The figure shows three views and two pictorial views of one solid part (mm, origin at its lowest corner). Answer the questions. A direction names the side the tool comes from. Coordinates: 2 decimals unless noted, no trailing zeros. Write each loop counter-clockwise with the first axis right and the second up, starting at its lowest first coordinate (ties: lowest second). Pieces come first, ordered by that corner, then holes.
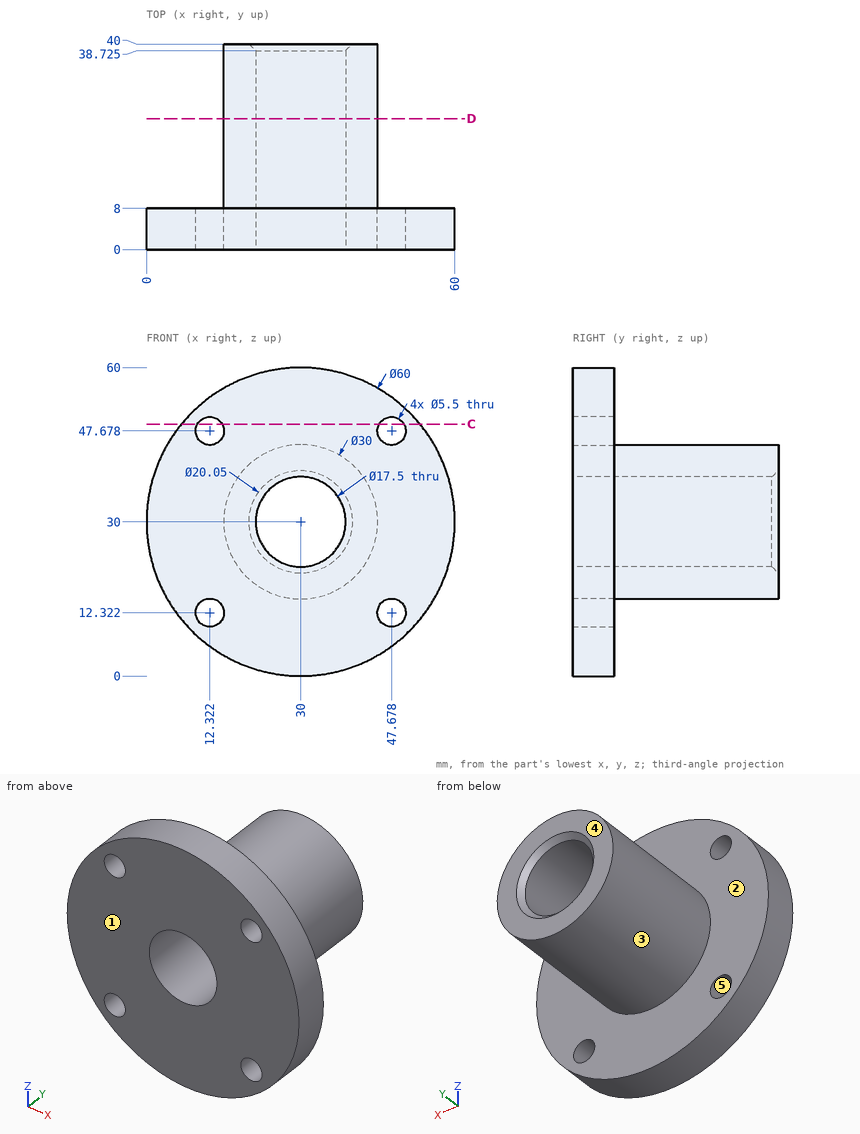
Q1. Which of the six approach directions +Z, -Z, +X, -X, +Y, -Y give full straight-line access (tool end or side, diameter ignored) to the marked faces 1 and 2?
Answers below:
face 1: +Z, -Z, +X, -X, -Y
face 2: +Y
Q2. The part is cut by section C-C, the plane z = 49. Write down the section's boundary in (x, y).
Answers below:
outline: (6.78, 0) - (9.91, 0) - (9.91, 8) - (6.78, 8) - close; (14.73, 0) - (45.27, 0) - (45.27, 8) - (14.73, 8) - close; (50.09, 0) - (53.22, 0) - (53.22, 8) - (50.09, 8) - close
Q3. Determine the mould class of the marked faces 3, 4 and 5 for opening direction X: released by +X, released by -X, zero draft, split by the parting line, or undercut.
Answers below:
face 3: split by the parting line
face 4: zero draft
face 5: undercut
Q4. Given pin 1 (5 mm diameter, centred on y = 29, z = 41, fed in from +X); pin 2 (4.5 mm diameter, centred on x = 47.68, z = 47.68, fed in from -Y); pin 3 (2 mm diameter, centred on x = 46.5, z = 36.5, fed in from +Y); pin 4 (8 mm diameter, centred on x = 30, y = 12.5, fed in from +Z), each flat-ended and moving along its own axis, determine where each tip first touches the part or whether it passes through.
Answers below:
pin 1: stops at x = 42.36
pin 2: passes through
pin 3: stops at y = 8
pin 4: stops at z = 45
Q5. Find the intervals of material crossed by probe 1 along Y at (x, z) = (49.5, 25); probe 2 along X at (y, z) = (26, 36); probe 3 along Z at (x, y) = (27.5, 7.5) (1 decimal), in increasing order.
Answers below:
probe 1: y = 0 to 8
probe 2: x = 16.25 to 23.63, 36.37 to 43.75
probe 3: z = 0.1 to 21.6, 38.4 to 59.9
Q6. The part is cut by section D-D, the plane y = 25.5. Write down the section's boundary in (x, z), then the cut area to 3 significant figures.
Answers below:
outline: circle Ø30 at (30, 30); hole circle Ø17.5 at (30, 30)
area: 466 mm2
